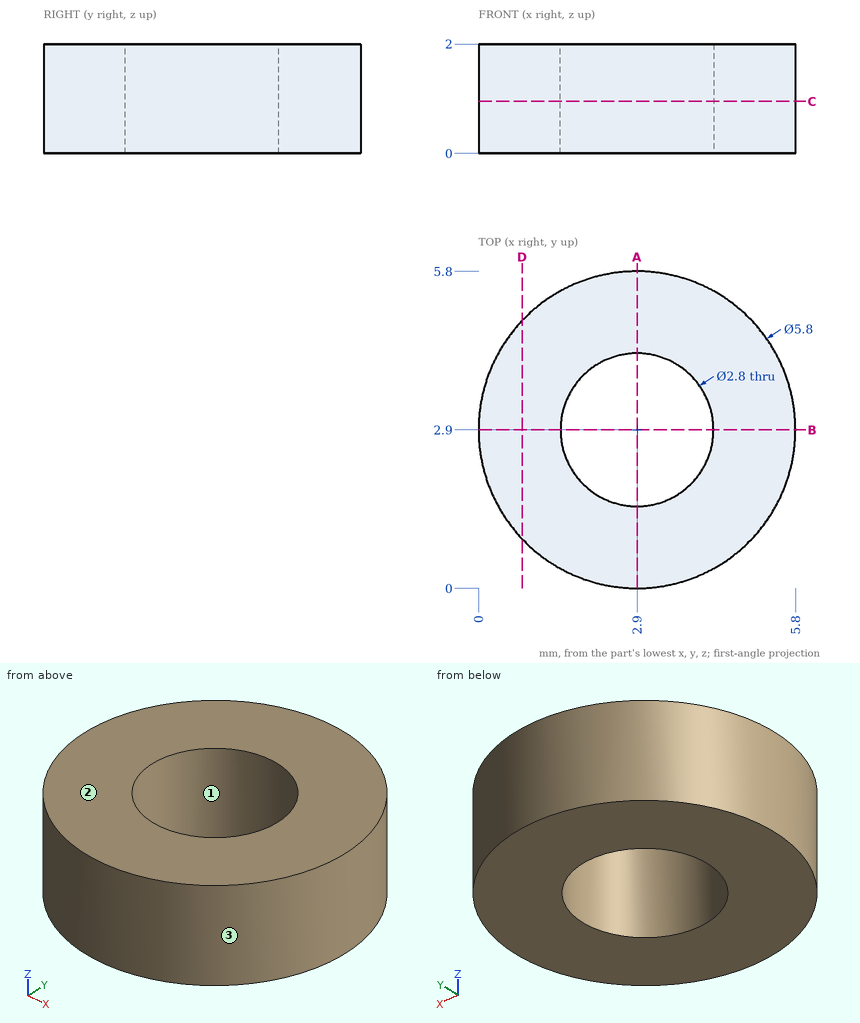
Source: three-view drawing plus pictorial views. Frame: mm from the lowest corner of the part. Give positions to 0.01 mm unless a question says otherwise; leave off trailing zeros. Loops run counter-clockwise (first coordinate to the right, second up) from the corner with the lowest first, then second, coordinate; pieces in that order, holes last. Notation, with made-up numbers: (-3, 62) -> (12, 62) arc R20 cw to (12, 83) -> close; hole circle Ø6 at (81.5, -23). An arc over 180 degrees is marked (long way). Use a Markdown table: item, result. Add a question column.
(1) Ray query, line 1 (Y direction, x = 2.9, z = 0.5); line 2 (X direction, y = 2.25, z = 1.15); line 3 (X direction, y = 2.05, z = 0.3). Return the intervals inside material, ascending.
(2) Section query A-A (x = 2.9). Output: boundary loops of the cut face in (y, z), then the cut area to 3 significant figures.
(3) Pull-direction query (X, two-part tool) for the marked faces 1, 2 and 3; classes: +X half, -X half, draft (parallel to the pull), parting line (faces both ways), or undercut.
(4) Section query D-D (x = 0.8). Output: boundary loops of the cut face in (y, z).
(5) Section query C-C (z = 0.95). Output: boundary loops of the cut face in (x, y), then the cut area to 3 significant figures.
Checked values:
| question | item | result |
|---|---|---|
| 1 | line 1 | 0 to 1.5, 4.3 to 5.8 |
| 1 | line 2 | 0.07 to 1.66, 4.14 to 5.73 |
| 1 | line 3 | 0.13 to 1.79, 4.01 to 5.67 |
| 2 | outline | (0, 0) -> (1.5, 0) -> (1.5, 2) -> (0, 2) -> close; (4.3, 0) -> (5.8, 0) -> (5.8, 2) -> (4.3, 2) -> close |
| 2 | area | 6.00 mm^2 |
| 3 | face 1 | undercut |
| 3 | face 2 | draft |
| 3 | face 3 | parting line |
| 4 | outline | (0.9, 0) -> (4.9, 0) -> (4.9, 2) -> (0.9, 2) -> close |
| 5 | outline | circle Ø5.8 at (2.9, 2.9); hole circle Ø2.8 at (2.9, 2.9) |
| 5 | area | 20.3 mm^2 |
